Design review of the part built by this model. Coordinates are the model's own, in mm. Face numbers are marked on the shaded views. A direction names the side the tool comes from. Coordinates: 2 decimals unless noted, no trailing zeros. Order: outer loops, then holes, each group sorted by start corner. A loop starts at its lowest first (then second) coordinate and runs counter-clockwise, first axis right, second up. Notation, with made-up numbers: M 51.5,28.25 L 105.5,28.25 A8 ccw 105.5,36.25 Z; hole C 48.5,36 d3. An arc over 180 degrees is marked long. Use CSV: the item, a comma, the result in double quotes.
```python
from build123d import *

# Parameters (mm, degrees)
F1_DEPTH = 14
F3_D     = 5.1


with BuildPart() as f1:
    # F0 (on Top) → F1 (new body)
    with BuildSketch(Plane.XY):
        with BuildLine():
            Line((-68.451825, 6.676397), (-68.451825, 0))
            Line((-68.451825, 0), (-26.451825, 0))
            Line((-26.451825, 0), (-26.451825, 6.846438))
            Line((-26.451825, 6.846438), (-37.451825, 6.846438))
            Line((-37.451825, 6.846438), (-37.451825, 37.5))
            Line((-37.451825, 37.5), (-45.951825, 37.5))
            Line((-45.951825, 37.5), (-45.951825, 28.809475))
            ThreePointArc((-45.951825, 28.809475), (-47.451825, 17), (-48.951825, 28.809475))
            Line((-48.951825, 28.809475), (-48.951825, 37.5))
            Line((-48.951825, 37.5), (-57.451825, 37.5))
            Line((-57.451825, 37.5), (-57.451825, 6.676397))
            Line((-57.451825, 6.676397), (-68.451825, 6.676397))
        make_face()
    extrude(amount=F1_DEPTH)

    # F3 (through all)
    with Locations(Plane.XZ):
        with Locations((-62.951825, 7), (-31.951825, 7)):
            Hole(F3_D / 2)


solid = f1.part
```
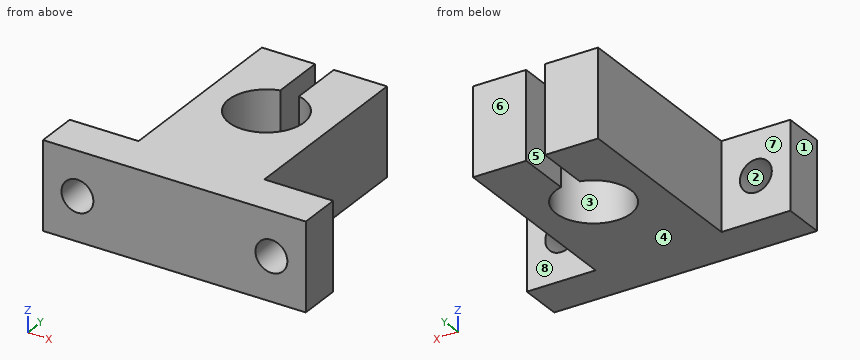
(1) Wall thickness on probe 1 along Y at (x, z) = (-35, 13); probe 2 along X at (y, z) = (15.5, 13.5); probe 3 along Y at (x, z) = (-50.5, 11.75): over which ranges is each line inside the solid? List them lowest first.
The answers:
probe 1,"y = 0 to 6.85"
probe 2,"x = -57.45 to -37.45"
probe 3,"y = 0 to 17.83, 28.17 to 37.5"
(2) Add section A-A on z = 7. State the section outline as (x, y) points, and give its area (3 significant figures).
The answers:
outline,"M -68.45,0 L -65.5,0 L -65.5,6.68 L -68.45,6.68 Z; M -60.4,0 L -34.5,0 L -34.5,6.85 L -37.45,6.85 L -37.45,37.5 L -45.95,37.5 L -45.95,28.81 A6 cw long -48.95,28.81 L -48.95,37.5 L -57.45,37.5 L -57.45,6.68 L -60.4,6.68 Z; M -29.4,0 L -26.45,0 L -26.45,6.85 L -29.4,6.85 Z"
area,"691 mm2"
(3) Add section B-B on y = 23. State the section outline as (x, z) points, and give its area (3 significant figures).
The answers:
outline,"M -57.45,0 L -53.45,0 L -53.45,14 L -57.45,14 Z; M -41.45,0 L -37.45,0 L -37.45,14 L -41.45,14 Z"
area,"112 mm2"
(4) Add section C-C on x = -43.5. State the section outline as (y, z) points, and give its area (3 significant figures).
The answers:
outline,"M 0,0 L 18.49,0 L 18.49,14 L 0,14 Z; M 27.51,0 L 37.5,0 L 37.5,14 L 27.51,14 Z"
area,"399 mm2"
(5) Clearance check with flat-ended pins moving along their axes: P1, Ø5.5, axis at x = -61.5, z = 8, coming from the +Y side; P2, Ø7, axis at x = -47.45, y = 23, coming from the +Z side; P3, Ø3, axis at y = 14.5, z = 9, coming from the -X side; P4, Ø2, axis at y = 22.5, z = 2.5, coming from the +X side. State where each tip first meets the part, or that it passes through.
The answers:
P1,"stops at y = 6.68"
P2,"passes through"
P3,"stops at x = -57.45"
P4,"stops at x = -37.45"
(6) The part is to be moulded in two halves that separate along X. For the marked faces 1, 2, 3 and 4, say which applies: pulls with the +X half, pulls with the -X half, needs draft (parallel to the pull), parting line crosses it, or undercut.
The answers:
face 1,"pulls with the -X half"
face 2,"undercut"
face 3,"undercut"
face 4,"needs draft"
(7) For the marked faces 5, 6, 7 and 8, list the 3-axis set-ups (+Z, -Z, +X, -X, +Y, -Y) from which the entire face can be reached by the end or side of a thin tool; tool diameter is ignored.
The answers:
face 5,"+Z, -Z, +Y"
face 6,"+Z, -Z, +X, -X, +Y"
face 7,"+Z, -Z, -X, +Y"
face 8,"+Z, -Z, +X, +Y"
(8) Add section D-D on z = 1.75. State the section outline as (x, y) points, and give its area (3 significant figures).
The answers:
outline,"M -68.45,0 L -26.45,0 L -26.45,6.85 L -37.45,6.85 L -37.45,37.5 L -45.95,37.5 L -45.95,28.81 A6 cw long -48.95,28.81 L -48.95,37.5 L -57.45,37.5 L -57.45,6.68 L -68.45,6.68 Z"
area,"760 mm2"
